Design review of the part built by this model. Coordinates are the model's own, in mm. A direction names the side the tool comes from. Coordinates: 2 decimals unless noted, no trailing zeros. Write each loop counter-clockwise with the first axis right and the second up, starting at its lowest first coordinate (ties: lowest second). Pieces come first, ordered by that corner, then holes. Notation, with made-up numbers: (35, 42.25) -> (77, 42.25) arc R19 cw to (77, 47.25) -> close; hole circle Ø3 at (31.5, 3.5). An arc over 180 degrees is marked (long way). Answer in a Markdown table with one row per item. Add a question column.
Item 1: Clearance check with a flat-ended pin moving along its axis: P1, Ø1.9, axis at x = -19.05, y = 0, coming from the -Z side. State where the tip first meets the part, or that it passes through.
Item 2: To check wall thickness, follow line 1 (X direction, y = 1.8, z = 3.75); line 2 (Y direction, x = -19.05, z = 0.45); line 3 (Z direction, x = -2, y = -0.25). State the ranges of each line that lie inside material, in increasing order.
Item 3: Draft analysis for pull direction Y (two halves, no side actions). For faces 1 (the face through (-0.2, 2.456, 0.3)), 2 (the face through (48.412, 0, 1)), 3 (the face through (44.84, 0.05, 0.4)), state which applies: released by +Y, released by -Y, zero draft, split by the parting line, or undercut.
Item 4: Take a section at A-A, the plane y = 0. Give the number of separate pieces and of enclosed holes in the cut face, and give its area (3 significant figures).
Item 5: For faces 4 (the face through (-1, 0, 0)), 5 (the face through (47.619, 0, 4)), list the 3-axis set-ups (+Z, -Z, +X, -X, +Y, -Y) from which the entire face can be reached by the end or side of a thin tool; tool diameter is ignored.
Item 6: Take a section at C-C, the plane x = -42. Write out the cut boundary in (y, z), and give its area (3 significant figures).
Item 7: Take a section at B-B, the plane x = -19.05. Write out the cut boundary in (y, z).
from build123d import *

# Parameters (mm, degrees)
SKETCH1_W           = 96.825
SKETCH1_H           = 4.9125
BOSS_EXTRUDE1_DEPTH = 4.9125
SHELL1_T            = -0.79375
SKETCH2_R           = 1.190625
CUT_EXTRUDE1_DEPTH  = 49.649433932
SKETCH3_R           = 1.190625
CUT_EXTRUDE2_DEPTH  = 97.98064985


with BuildPart() as part:
    # Sketch1 → Boss-Extrude1 (new body)
    with BuildSketch(Plane.XY):
        Rectangle(SKETCH1_W, SKETCH1_H)
    extrude(amount=BOSS_EXTRUDE1_DEPTH)

    # Shell1
    shell1_openings = [part.faces().sort_by_distance(p)[0] for p in [
        (0, 0, 4.9125),
        (0, -2.45625, 2.45625),
        (0, 2.45625, 2.45625),
    ]]
    offset(amount=SHELL1_T, openings=shell1_openings, kind=Kind.INTERSECTION)

    # Sketch2 → Cut-Extrude1 (cut, through all)
    with BuildSketch(Plane.XY.offset(0.79375)):
        with Locations((-46.03125, 0)):
            Circle(SKETCH2_R)
        with Locations((-19.05, 0)):
            Circle(SKETCH2_R)
        with Locations((19.05, 0)):
            Circle(SKETCH2_R)
        with Locations((46.03125, 0)):
            Circle(SKETCH2_R)
    extrude(amount=-CUT_EXTRUDE1_DEPTH, mode=Mode.SUBTRACT)

    # Sketch3 → Cut-Extrude2 (cut, through all)
    with BuildSketch(Plane.ZY.offset(48.4125)):
        with Locations((2.53125, 0)):
            Circle(SKETCH3_R)
    extrude(amount=-CUT_EXTRUDE2_DEPTH, mode=Mode.SUBTRACT)


solid = part.part
Answers:
| question | item | result |
|---|---|---|
| 1 | P1 | passes through |
| 2 | line 1 | x = -48.41 to -47.62, 47.62 to 48.41 |
| 2 | line 2 | y = -2.46 to -1.19, 1.19 to 2.46 |
| 2 | line 3 | z = 0 to 0.79 |
| 3 | face 1 | released by +Y |
| 3 | face 2 | zero draft |
| 3 | face 3 | undercut |
| 4 | separate pieces | 7 |
| 4 | enclosed holes | 0 |
| 4 | area | 72.1 mm^2 |
| 5 | face 4 | -Z, +X, -X, +Y, -Y |
| 5 | face 5 | +Z, +Y, -Y |
| 6 | outline | (-2.46, 0) -> (2.46, 0) -> (2.46, 0.79) -> (-2.46, 0.79) -> close |
| 6 | area | 3.90 mm^2 |
| 7 | outline | (-2.46, 0) -> (-1.19, 0) -> (-1.19, 0.79) -> (-2.46, 0.79) -> close; (1.19, 0) -> (2.46, 0) -> (2.46, 0.79) -> (1.19, 0.79) -> close |
